Part model, mm, in its own coordinate system. Round coordinates to 2 decimals unless told otherwise and drop trailing zeros. Write each loop counter-clockwise with the first axis right and the second up, starting at its lowest first coordinate (ties: lowest second). Pieces come first, ordered by that corner, then holes. Notation, with made-up numbers: (12, -22) -> (22, -22) arc R11 cw to (22, -16) -> close; hole circle Ø5 at (-11.75, -23). An arc over 180 degrees is marked (long way). Return JSON: item names as keys, results as strings. Group by question number.
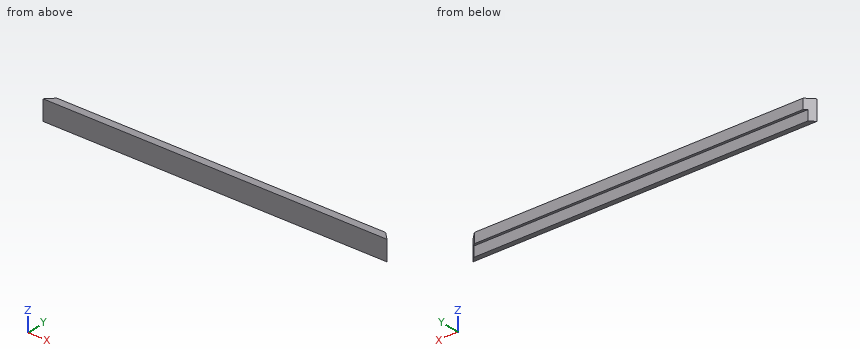
```python
from build123d import *

# Parameters (mm, degrees)
F0_W     = 762
F0_H     = 50.8
F1_DEPTH = 19.05
F3_DEPTH = 762.001
F4_DEPTH = 50.8
F5_DEPTH = 50.8
F7_DEPTH = 50.801


with BuildPart() as f1:
    # F0 (on Front) → F1 (new body)
    with BuildSketch(Plane.XZ):
        Rectangle(F0_W, F0_H)
    extrude(amount=F1_DEPTH)

    # F2 (on face) → F3 (cut, through all)
    with BuildSketch(Plane(origin=(-381, 0, 0), x_dir=(0, -1, 0), z_dir=(-1, 0, 0))):
        Polygon((6.35, -29.9884248525), (6.35, -25.4), (6.35, 0), (0, 0), (-13.0046028644, 0), (-13.0046028644, -29.9884248525), align=None)
    extrude(amount=-F3_DEPTH, mode=Mode.SUBTRACT)

    # F4 (add): a face of the model
    f4_faces = [f1.faces().sort_by_distance(p)[0] for p in [
        (-381, -10.795, 2.54),
    ]]
    extrude(f4_faces, amount=F4_DEPTH)

    # F5 (add): a face of the model
    f5_faces = [f1.faces().sort_by_distance(p)[0] for p in [
        (381, -10.795, 2.54),
    ]]
    extrude(f5_faces, amount=F5_DEPTH)

    # F6 (on face) → F7 (cut, through all)
    with BuildSketch(Plane.XY.offset(25.4)):
        Polygon((412.75, 0), (431.8, -19.05), (436.4477694035, -19.05), (436.4477694035, 9.3147736043), (412.75, 9.3147736043), align=None)
        Polygon((-444.389373064, -19.05), (-431.8, -19.05), (-412.75, 0), (-412.75, 9.4755124301), (-444.389373064, 9.4755124301), align=None)
    extrude(amount=-F7_DEPTH, mode=Mode.SUBTRACT)


solid = f1.part
```
Item 1: Cut at A-A (y = -11.25). Write the cut outline in (x, z), then the cut area to 3 significant figures.
Item 2: Wall check: L1, parallel to Z at x = -196, y = -1.75; L2, parallel to Y at x = -238, z = -9; L3, parallel to X at y = -9.25, z = 0. Give the ranges that are in metal, low to high.
Item 3: Cut at B-B (x = -350). Write the cut outline in (y, z), then the cut area to 3 significant figures.
Item 4: Cut at C-C (z = -9.5). Write the cut outline in (x, y).
Item 5: Flat gauge pins, fed straight in: P1, Ø1.9, axis at x = 192, y = -2.5, coming from the -Z side; P2, Ø5, axis at x = -63.5, z = -13, coming from the +Y side; P3, Ø5, axis at y = -13, z = -10.5, coming from the -X side. Where does each tip first touch, or does it go through?
Checks:
{
 "1": {"outline": "(-424, -25.4) -> (424, -25.4) -> (424, 25.4) -> (-424, 25.4) -> close", "area": "43,100 mm2"},
 "2": {"L1": "z = 0 to 25.4", "L2": "y = -19.05 to -6.35", "L3": "x = -422 to 422"},
 "3": {"outline": "(-19.05, -25.4) -> (-6.35, -25.4) -> (-6.35, 0) -> (0, 0) -> (0, 25.4) -> (-19.05, 25.4) -> close", "area": "806 mm2"},
 "4": {"outline": "(-431.8, -19.05) -> (431.8, -19.05) -> (419.1, -6.35) -> (-419.1, -6.35) -> close"},
 "5": {"P1": "stops at z = 0", "P2": "stops at y = -6.35", "P3": "stops at x = -428.25"}
}
